Print and shaded views of the part. All mm, measured from the part's lowest x, y and z. A direction names the side the tool comes from. Give positions to 0.01 mm unless a question says otherwise; leave off trailing zeros. Order: outer loops, then holes, each group sorted by start corner. A loop starts at its lowest first (then second) coordinate and runs counter-clockwise, first axis right, second up. Notation, with made-up numbers: (-11, -28) - (40, -28) arc R24 ccw to (40, -3) - close; hole circle Ø10 at (47.5, 20). An arc over 180 degrees is marked (long way). Answer in a Markdown table with one row per item.
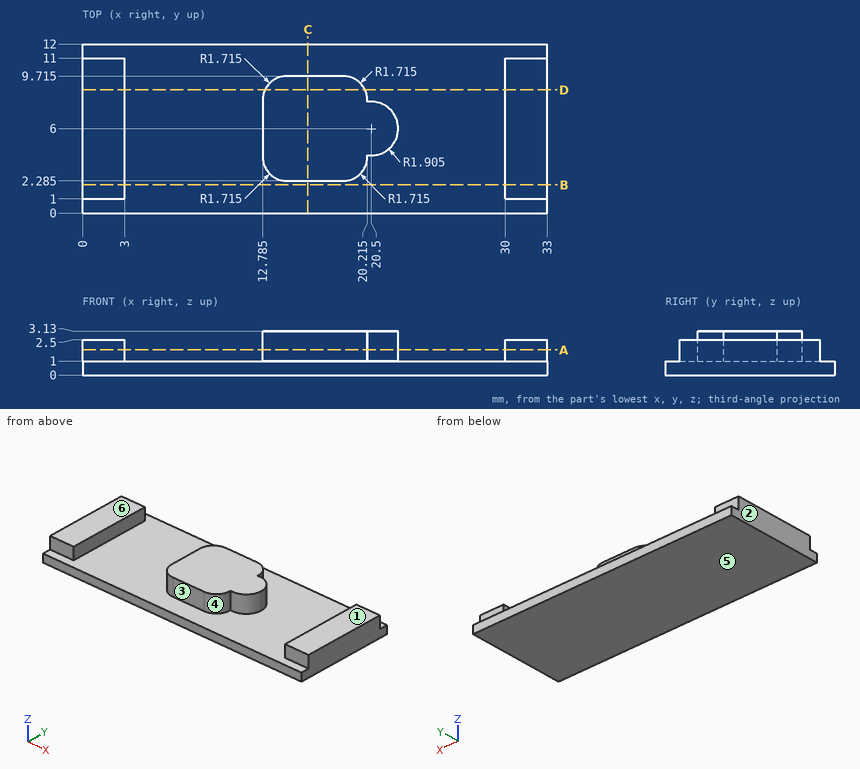
1. Cut at B-B on y = 2. Write the cut outline in (x, z).
Check result:
| item | result |
|---|---|
| outline | (0, 0) - (33, 0) - (33, 2.5) - (30, 2.5) - (30, 1) - (3, 1) - (3, 2.5) - (0, 2.5) - close |
2. Drop flat-ended pins along their axis: P1, Ø3.5, axis at x = 31.5, y = 7.5, coming from the +Z side; P2, Ø1.1, axis at x = 15.5, z = 2.5, coming from the +Y side (1 decimal); P3, Ø1.1, axis at x = 16.5, z = 2, coming from the -Y side (1 decimal). Give the stop position or say it passes through.
Check result:
| item | result |
|---|---|
| P1 | stops at z = 2.5 |
| P2 | stops at y = 9.7 |
| P3 | stops at y = 2.3 |
3. Cut at A-A on z = 1.8. Count the separate pieces of the cut face and the enclosed holes in it.
Check result:
| item | result |
|---|---|
| separate pieces | 3 |
| enclosed holes | 0 |
4. Cut at D-D on y = 8.75. Write the cut outline in (x, z).
Check result:
| item | result |
|---|---|
| outline | (0, 0) - (33, 0) - (33, 2.5) - (30, 2.5) - (30, 1) - (20.04, 1) - (20.04, 3.13) - (12.96, 3.13) - (12.96, 1) - (3, 1) - (3, 2.5) - (0, 2.5) - close |
5. Cut at C-C on x = 16. Write the cut outline in (y, z) (1 decimal).
Check result:
| item | result |
|---|---|
| outline | (0, 0) - (12, 0) - (12, 1) - (9.7, 1) - (9.7, 3.1) - (2.3, 3.1) - (2.3, 1) - (0, 1) - close |
6. Probe line 1 (X direction, y = 8, z = 1.9) (1 decimal); line 2 (X direction, y = 2, z = 2.15); line 3 (X direction, y = 8.5, z = 1.15). List the from-to ranges inside material, lowest first.
Check result:
| item | result |
|---|---|
| line 1 | x = 0 to 3, 12.8 to 20.2, 30 to 33 |
| line 2 | x = 0 to 3, 30 to 33 |
| line 3 | x = 0 to 3, 12.86 to 20.14, 30 to 33 |
7. Which spindle directions (+Z, -Z, +X, -X, +Y, -Y) get a long thin tool onto all of the face, cutting with end or side? Do the marked faces 5 and 6. Say none if no direction does.
Check result:
| item | result |
|---|---|
| face 5 | -Z, +X, -X, +Y, -Y |
| face 6 | +Z, -X, +Y, -Y |
8. Two-plate mould, pull along X, no slides. Class the marked faces 1, 2, 3 and 4: +X half, -X half, draft (parallel to the pull), parting line (faces both ways), or undercut.
Check result:
| item | result |
|---|---|
| face 1 | draft |
| face 2 | -X half |
| face 3 | undercut |
| face 4 | undercut |
